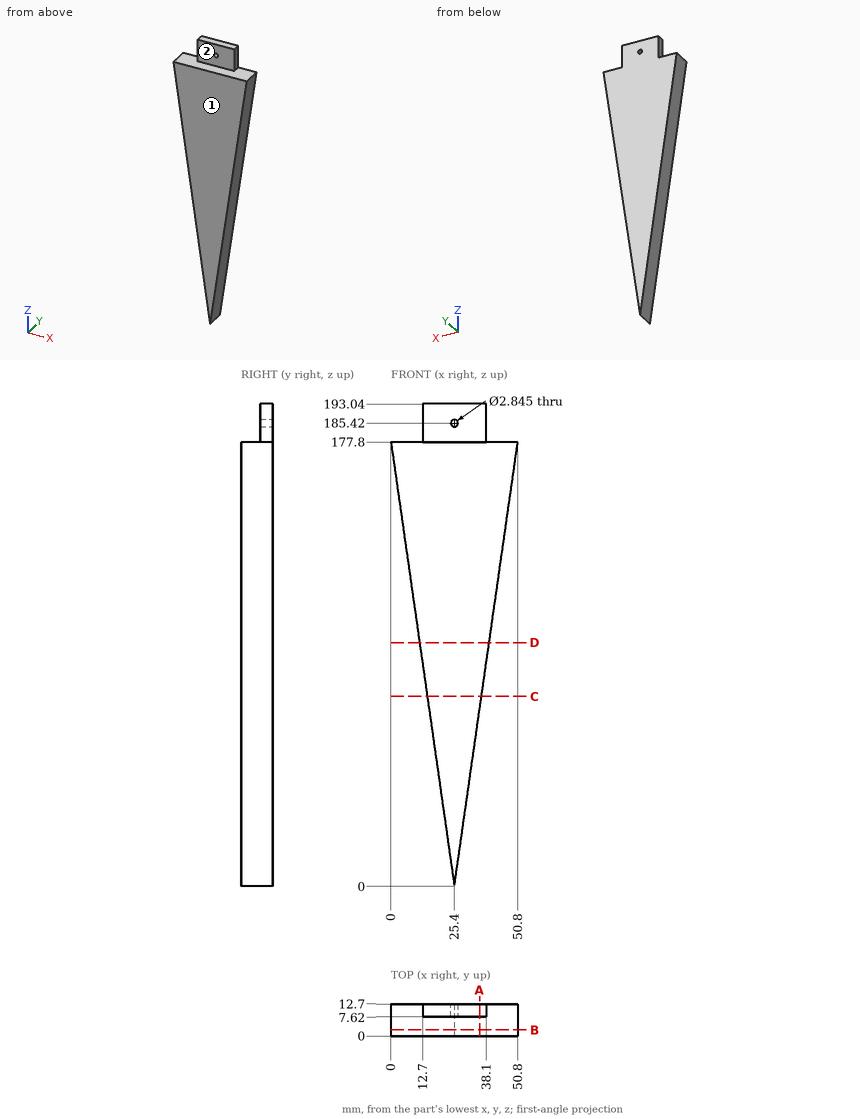
Can you work these out from the drawing? Everything is in mm from the part's minimum corner. A direction names the side the tool comes from. Coordinates: 2 decimals unless noted, no trailing zeros. Order: outer loops, then holes, each group sorted by start corner. A loop starts at its lowest first (then second) coordinate and runs counter-clockwise, first axis right, second up. Notation, with made-up numbers: (-6.5, 73) -> (30.5, 73) arc R24 ccw to (30.5, 85) -> close; hole circle Ø4 at (68.5, 58.25). An arc over 180 degrees is marked (long way). Use one line per item in the form item = value.
Q1. Imagine slicing it at A-A, the plane x = 35.5. List the corners of the cut face in (y, z) for me, then the cut area to 3 significant figures.
From the geometry:
outline = (0, 70.7) -> (12.7, 70.7) -> (12.7, 193.04) -> (7.62, 193.04) -> (7.62, 177.8) -> (0, 177.8) -> close
area = 1,440 mm²
Q2. Will these pins go through, and if not, where does the flat tip stop? P1, Ø6, axis at y = 6.5, z = 63, coming from the +X side; P2, Ø2, axis at y = 8.5, z = 58, coming from the +X side; P3, Ø5, axis at y = 9.5, z = 30.5, coming from the -X side.
From the geometry:
P1 = 34.83
P2 = 33.83
P3 = 20.69
Q3. Imagine slicing it at C-C, the plane z = 76. List the corners of the cut face in (x, y) for me, then the cut area to 3 significant figures.
From the geometry:
outline = (14.54, 0) -> (36.26, 0) -> (36.26, 12.7) -> (14.54, 12.7) -> close
area = 276 mm²
Q4. Imagine slicing it at D-D, the plane z = 97.5. List the corners of the cut face in (x, y) for me.
From the geometry:
outline = (11.47, 0) -> (39.33, 0) -> (39.33, 12.7) -> (11.47, 12.7) -> close
Q5. Imagine slicing it at B-B, the plane y = 2.5. List the corners of the cut face in (x, z) for me, then the cut area to 3 significant figures.
From the geometry:
outline = (0, 177.8) -> (25.4, 0) -> (50.8, 177.8) -> close
area = 4,520 mm²
Q6. I need wall thicknesses on L1, parallel to X at y = 4.25, z = 37; L2, parallel to X at y = 6.25, z = 122.5. Which ranges of each line are inside material? Lowest first, please.
From the geometry:
L1 = 20.11 to 30.69
L2 = 7.9 to 42.9
Q7. Which directions (+Z, -Z, +X, -X, +Y, -Y) give clear straight access to the entire face, cutting with the end or side of a thin tool? Please do the marked faces 1 and 2.
From the geometry:
face_1 = +Z, -Z, +X, -X, -Y
face_2 = +Z, +X, -X, -Y
